For this review, take the finished solid that the model builds, in its own axes (mm). A direction names the side the tool comes from. Give positions to 0.01 mm unless a question says otherwise; leave off trailing zeros. Order: outer loops, then holes, each group sorted by start corner. A loop starts at its lowest first (then second) coordinate and runs counter-clockwise, first axis right, second up. Notation, with made-up numbers: M 59,78.25 L 116,78.25 A27 ccw 116,99.25 Z; hole C -5.5,48 d2. An arc over 180 degrees is marked long. Answer as CSV lines item,"result". Start each with the question number.
1. We need section B-B, the plane y = 0. Give the boundary of the cut face in (x, z).
2. Clearance check with a flat-ended pin moving along its axis: P1, Ø9, axis at x = 52.5, y = 90.93, coming from the -Z side. State where the tip first meets the part, or that it passes through.
3. For line 1 along X through (y, z) = (-1.5, 7.5); line 2 along Y through (x, z) = (-52.5, 9); line 3 along Y through (x, z) = (-29, 10.75), list the stretches that pass through material, from the lowest coordinate up.
4. We need section A-A, the plane x = -107.5. Give the boundary of the cut face in (y, z).
5. Machinability: for faces 1 (the flat face through (-88, 31, 22)), 2 (the flat face through (116, -102, 11)), which of the approach directions +Z, -Z, +X, -X, +Y, -Y give a long, thin tool a straight path to every point of the face, cutting with its end or side? Answer none if there is none.
6. We need section C-C, the plane x = -4. Give the boundary of the cut face in (y, z), and give its area (3 significant figures).
7. We need section D-D, the plane z = 7.5. State how many separate pieces and enclosed holes the cut face has, and give its area (3 significant figures).
8. Mouldability with a two-part tool opening along X and no side actions: class faces 3 (the cylindrical face through (95.797, 54.032, 10.846)), 4 (the flat face through (130, -2, 11)), 5 (the cylindrical face through (-125.72, -125.49, 11.15)) as pulls with the +X half, pulls with the -X half, needs draft (parallel to the pull), parting line crosses it, or undercut.
from build123d import *

# Parameters (mm, degrees)
SKETCH_1_W               = 260
SKETCH_1_H               = 260
EXTRUDE_1_DEPTH          = 22
FILLET_1_R               = 15
CUT_EXTRUDE_1_DEPTH      = 186.159390796
CUT_EXTRUDE_1_DEPTH_BACK = 186.159390796
SKETCH_2_R               = 92.5
SKETCH_2_R_2             = 5.1
CUT_EXTRUDE_2_DEPTH      = 186.159390796
CUT_EXTRUDE_2_DEPTH_BACK = 186.159390796


with BuildPart() as part:
    # ｽｹｯﾁ1 → ﾎﾞｽ - 押し出し1 (new body)
    with BuildSketch(Plane.XY):
        Rectangle(SKETCH_1_W, SKETCH_1_H)
    extrude(amount=EXTRUDE_1_DEPTH)

    # ﾌｨﾚｯﾄ1
    fillet_1_edges = [part.edges().sort_by_distance(p)[0] for p in [
        (-130, 130, 11),
        (130, 130, 11),
        (130, -130, 11),
        (-130, -130, 11),
    ]]
    fillet(fillet_1_edges, radius=FILLET_1_R)

    # ｽｹｯﾁ2 → ｶｯﾄ - 押し出し1 (cut, two sides: drawn at the far end of the back side and taken through both)
    with BuildSketch(Plane.XY.offset(-CUT_EXTRUDE_1_DEPTH_BACK)):
        Circle(SKETCH_2_R)
        with Locations((90.932667397, 52.5)):
            Circle(SKETCH_2_R_2)
        with Locations((52.5, 90.932667397)):
            Circle(SKETCH_2_R_2)
        with Locations((-52.5, 90.932667397)):
            Circle(SKETCH_2_R_2)
        with Locations((-90.932667397, 52.5)):
            Circle(SKETCH_2_R_2)
        with Locations((-90.932667397, -52.5)):
            Circle(SKETCH_2_R_2)
        with Locations((-52.5, -90.932667397)):
            Circle(SKETCH_2_R_2)
        with Locations((52.5, -90.932667397)):
            Circle(SKETCH_2_R_2)
        with Locations((90.932667397, -52.5)):
            Circle(SKETCH_2_R_2)
    extrude(amount=CUT_EXTRUDE_1_DEPTH + CUT_EXTRUDE_1_DEPTH_BACK, mode=Mode.SUBTRACT)

    # ｽｹｯﾁ3 → ｶｯﾄ - 押し出し2 (cut, two sides: drawn at the far end of the back side and taken through both)
    with BuildSketch(Plane.XY.offset(-CUT_EXTRUDE_2_DEPTH_BACK)):
        with BuildLine():
            Line((-116, -107.5), (-116, -97.5))
            ThreePointArc((-116, -97.5), (-107.5, -89), (-99, -97.5))
            Line((-99, -97.5), (-99, -107.5))
            ThreePointArc((-99, -107.5), (-107.5, -116), (-116, -107.5))
        make_face()
        with BuildLine():
            Line((-116, 97.5), (-116, 107.5))
            ThreePointArc((-116, 107.5), (-107.5, 116), (-99, 107.5))
            Line((-99, 107.5), (-99, 97.5))
            ThreePointArc((-99, 97.5), (-107.5, 89), (-116, 97.5))
        make_face()
        with BuildLine():
            Line((99, -107.5), (99, -97.5))
            ThreePointArc((99, -97.5), (107.5, -89), (116, -97.5))
            Line((116, -97.5), (116, -107.5))
            ThreePointArc((116, -107.5), (107.5, -116), (99, -107.5))
        make_face()
        with BuildLine():
            Line((99, 97.5), (99, 107.5))
            ThreePointArc((99, 107.5), (107.5, 116), (116, 107.5))
            Line((116, 107.5), (116, 97.5))
            ThreePointArc((116, 97.5), (107.5, 89), (99, 97.5))
        make_face()
    extrude(amount=CUT_EXTRUDE_2_DEPTH + CUT_EXTRUDE_2_DEPTH_BACK, mode=Mode.SUBTRACT)


solid = part.part
Result set:
1,outline,"M -130,0 L -92.5,0 L -92.5,22 L -130,22 Z; M 92.5,0 L 130,0 L 130,22 L 92.5,22 Z"
2,P1,"through"
3,line 1,"-130 to -92.49, 92.49 to 130"
3,line 2,"-130 to -96.03, -85.83 to -76.16, 76.16 to 85.83, 96.03 to 130"
3,line 3,"-130 to -87.84, 87.84 to 130"
4,outline,"M -130,0 L -116,0 L -116,22 L -130,22 Z; M -89,0 L 89,0 L 89,22 L -89,22 Z; M 116,0 L 130,0 L 130,22 L 116,22 Z"
5,face 1,"+Z, +X, -X, +Y, -Y"
5,face 2,"+Z, -Z"
6,outline,"M -130,0 L -92.41,0 L -92.41,22 L -130,22 Z; M 92.41,0 L 130,0 L 130,22 L 92.41,22 Z"
6,area,"1,650 mm2"
7,separate pieces,"1"
7,enclosed holes,"13"
7,area,"38,300 mm2"
8,face 3,"undercut"
8,face 4,"pulls with the +X half"
8,face 5,"pulls with the -X half"
